from build123d import *

# Parameters (mm, degrees)
CHANFRO1_SIZE = 0.5


with BuildPart() as part:
    # Esboço1 → Revolução1 (revolve)
    with BuildSketch(Plane(origin=(0, 0, 0), x_dir=(1, 0, 0), z_dir=(0, 1, 0)), mode=Mode.PRIVATE) as revolu_o1_sk:
        Polygon((0, 0), (0, 11), (-20, 11), (-20, 9), (-47, 9), (-47, 8.5), (-48.3, 8.5), (-48.3, 9), (-50, 9), (-50, 0), align=None)
    revolve(revolu_o1_sk.sketch.rotate(Axis((-50, 0, 0), (1, 0, 0)), 180), axis=Axis((-50, 0, 0), (1, 0, 0)))

    # Chanfro1
    chanfro1_edges = [part.edges().sort_by_distance(p)[0] for p in [
        (-50, 0, -9),
    ]]
    chamfer(chanfro1_edges, length=CHANFRO1_SIZE)


solid = part.part
Input: part model. Units: mm. Frame: model coordinates. A direction names the side the tool comes from. Coordinates: 2 decimals unless noted, no trailing zeros. Loops run counter-clockwise (first coordinate to the right, second up) from the corner with the lowest first, then second, coordinate; pieces in that order, holes last.
Q1. Draft query along X for faces 1 (the face through (-47.659, -8.428, -1.107)), 2 (the face through (0, 0, 0)), 3 (the face through (-20, 9, 2)), 4 (the face through (-48.908, -6.083, -6.633)). Return one class per face: +X half, -X half, draft (parallel to the pull), parting line (faces both ways), or undercut.
Q2. Cut plane D-D (x = -21.5). Output: boundary loops of the cut face in (y, z).
Q3. Set-up query: faces 5 (the face through (-33.689, -6.083, -6.633)), 6 (the face through (-10.14, 10.74, -2.38)), 7 (the face through (-48.3, 3.3, -8)). Return all of +Z, -Z, +X, -X, +Y, -Y with unobstructed straight access to the full face (end or side cutting, diameter ignored); none if empty.
Q4. Contact query for flat-ended pins moving along their axis: pin 1 (2 mm diameter, centred on x = -43.5, z = 7.5, fed in from +Y); pin 2 (4 mm diameter, centred on x = -15, y = 1, fed in from +Z); pin 3 (12 mm diameter, centred on x = -32, z = -0.5, fed in from +Y); pin 4 (12 mm diameter, centred on x = -35, y = 0.5, fed in from +Z). Output: stop coordinate, or through.
Q5. Cut plane C-C (x = -8). Output: boundary loops of the cut face in (y, z).
Q6. Material intervals for line 1 (X direction, y = -6.5, z = -7.25); line 2 (Y direction, x = -10, z = 0.25); line 3 (Z direction, x = -2.5, y = -4.25), sorted ascending.
Q7. Cut plane A-A (y = 0). Output: boundary loops of the cut face in (x, z).
Working result:
1. face 1: undercut
1. face 2: +X half
1. face 3: -X half
1. face 4: draft
2. outline: circle Ø18 at (0, 0)
3. face 5: -X
3. face 6: +X, -X
3. face 7: none
4. pin 1: stops at y = 6.22
4. pin 2: stops at z = 11
4. pin 3: stops at y = 9
4. pin 4: stops at z = 9
5. outline: circle Ø22 at (0, 0)
6. line 1: x = -20 to 0
6. line 2: y = -11 to 11
6. line 3: z = -10.15 to 10.15
7. outline: (-50, -8.5) - (-49.5, -9) - (-48.3, -9) - (-48.3, -8.5) - (-47, -8.5) - (-47, -9) - (-20, -9) - (-20, -11) - (0, -11) - (0, 11) - (-20, 11) - (-20, 9) - (-47, 9) - (-47, 8.5) - (-48.3, 8.5) - (-48.3, 9) - (-49.5, 9) - (-50, 8.5) - close
